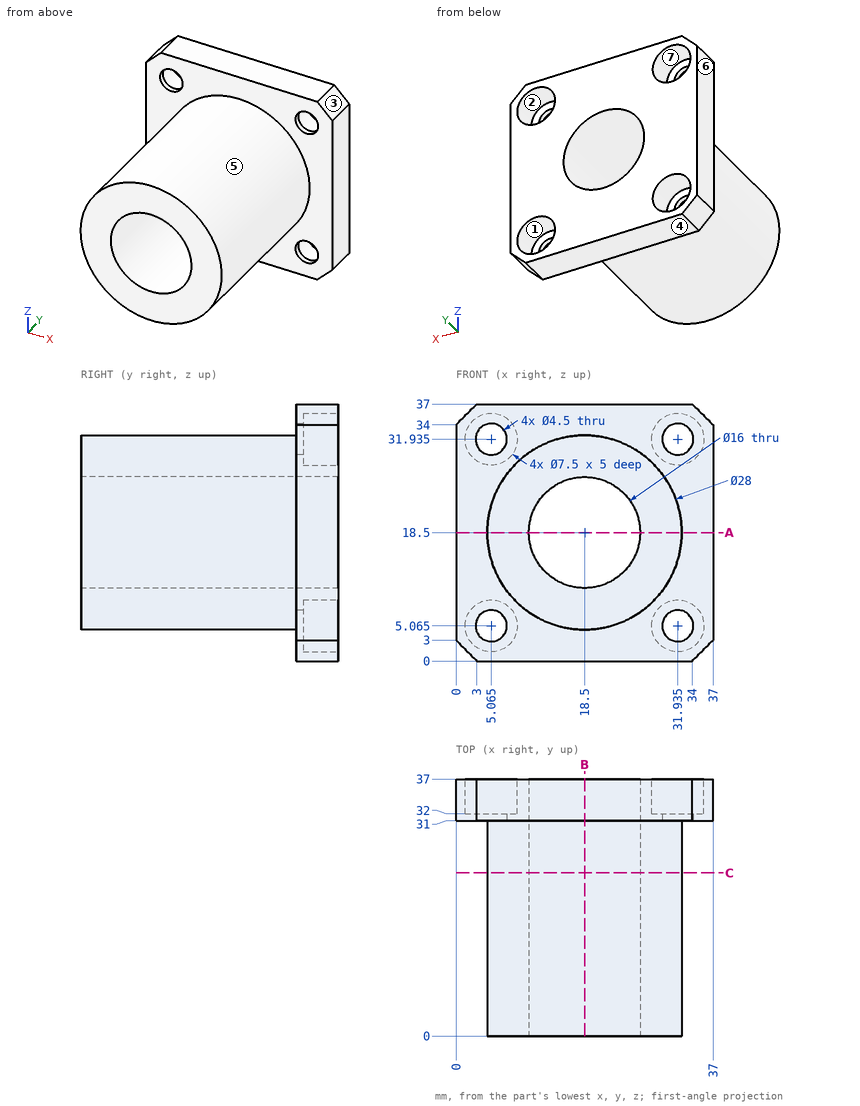
Input: dimensioned drawing with shaded views. Units: mm. Origin: part minimum x, y, z. A direction names the side the tool comes from. Give positions to 0.01 mm unless a question says otherwise; leave off trailing zeros. Order: outer loops, then holes, each group sorted by start corner. A loop starts at its lowest first (then second) coordinate and runs counter-clockwise, first axis right, second up. Notation, with made-up numbers: (12, 55) -> (67, 55) arc R33 cw to (67, 86) -> close; hole circle Ø8 at (80, -30.5). An arc over 180 degrees is marked (long way). Use a Markdown table: item, result.
1) Contact query for flat-ended pins moving along their axis: P1, Ø6, axis at x = 5.06, z = 5.06, coming from the +Y side; P2, Ø12, axis at x = 22.5, y = 4, coming from the -Z side; P3, Ø12, axis at y = 23, z = 29, coming from the +X side. Output: stop coordinate, or through.
Answer list:
| item | result |
|---|---|
| P1 | y = 32 |
| P2 | z = 4.5 |
| P3 | x = 31.76 |
2) Reachability of the marked faces 5, 6 and 7 from +Z, -Z, +X, -X, +Y, -Y: full face, straight path, thin tool, end or side. Return the list, or none.
Answer list:
| item | result |
|---|---|
| face 5 | -Y |
| face 6 | +Z, -Z, -X, +Y, -Y |
| face 7 | +Y |
3) Mould query, pull axis Z, two halves, no side actions, for the marked faces 1, 2, 3 and 4. Classes: +Z half, -Z half, draft (parallel to the pull), parting line (faces both ways), or undercut.
Answer list:
| item | result |
|---|---|
| face 1 | undercut |
| face 2 | undercut |
| face 3 | +Z half |
| face 4 | -Z half |
4) Section query B-B, the plane x = 18.5. Return the cut outline in (y, z).
Answer list:
| item | result |
|---|---|
| outline | (0, 4.5) -> (31, 4.5) -> (31, 0) -> (37, 0) -> (37, 10.5) -> (0, 10.5) -> close; (0, 26.5) -> (37, 26.5) -> (37, 37) -> (31, 37) -> (31, 32.5) -> (0, 32.5) -> close |
5) Section query A-A, the plane z = 18.5. Return the cut outline in (x, y).
Answer list:
| item | result |
|---|---|
| outline | (0, 31) -> (4.5, 31) -> (4.5, 0) -> (10.5, 0) -> (10.5, 37) -> (0, 37) -> close; (26.5, 0) -> (32.5, 0) -> (32.5, 31) -> (37, 31) -> (37, 37) -> (26.5, 37) -> close |
6) Ray query, line 1 along Z through (x, y) = (32.5, 31.5); line 2 along X through (y, z) = (15.5, 15.5); line 3 along X through (y, z) = (20.5, 13.5) (3 decimals). Return the intervals inside material, ascending. Write a range as [from, to].
Answer list:
| item | result |
|---|---|
| line 1 | [0, 2.89], [7.24, 29.76], [34.11, 37] |
| line 2 | [4.83, 11.08], [25.92, 32.17] |
| line 3 | [5.423, 12.255], [24.745, 31.577] |
7) Section query C-C, the plane y = 23.5. Return the cut outline in (x, z).
Answer list:
| item | result |
|---|---|
| outline | circle Ø28 at (18.5, 18.5); hole circle Ø16 at (18.5, 18.5) |
